The listing builds one solid part. Answer for the finished solid, in the listing's coordinates (mm). Round coordinates to 2 decimals unless told otherwise and drop trailing zeros. Loops run counter-clockwise (first coordinate to the right, second up) from the corner with the lowest first, then second, coordinate; pieces in that order, holes last. Notation, with made-up numbers: (50.5, -15) - (64.5, -15) arc R25 ccw to (64.5, 6) - close; hole circle Ø9 at (55.25, -29.75). An arc over 180 degrees is marked (long way). Write item = value, one per line. Start each with the question number.
1) Section C-C, the plane y = 5.4 is taken. Determine the outline of the cut face in (x, z), and give its area (3 significant figures).
2) Given pin 1 Ø10 at (x, z) = (-14, 16) entering from +Y; pin 2 Ø0.7 at (y, z) = (0.5, 1) entering from -X, each flat-ended and moving along its own axis, determine where each tip first touches the part or whether it passes through.
3) Section B-B, the plane x = -16.75 is taken. Determine the outline of the cut face in (y, z).
4) Section A-A, the plane y = 2.9 is taken. Determine the outline of the cut face in (x, z).
5) Section D-D, the plane x = -9.25 is taken. Determine the outline of the cut face in (y, z), and give its area (3 significant figures).
6) Straight lines are drawn through the part: line 1 along Z through (x, y) = (-11.5, 0.65); line 2 along X through (y, z) = (3.05, 26); line 3 along Y through (x, z) = (2, -10). For each, find the intervals that lie inside material, in ascending order.
from build123d import *

# Parameters (mm, degrees)
BOSS_EXTRUDE1_START       = -15.875
BOSS_EXTRUDE1_DEPTH       = 15.875
BOSS_EXTRUDE1_2_OUTLINE_W = 13.197490677
BOSS_EXTRUDE1_2_OUTLINE_H = 1.397
BOSS_EXTRUDE1_2_DEPTH     = 16.6878
SKETCH2_W                 = 13.197490677
SKETCH2_H                 = 1.397
BOSS_EXTRUDE2_DEPTH       = 16.6878
BOSS_EXTRUDE3_START       = 7.1247
BOSS_EXTRUDE3_DEPTH       = 7.1247
BOSS_EXTRUDE4_DEPTH       = 7.1247
CUT_EXTRUDE1_DEPTH        = 38.210837465
CUT_EXTRUDE2_DEPTH        = 38.210837465
CUT_EXTRUDE3_DEPTH        = 38.210837465
CUT_EXTRUDE4_DEPTH        = 38.210837465
SKETCH9_W                 = 4.6228
SKETCH9_H                 = 4.6228
CUT_EXTRUDE5_DEPTH        = 38.408183622
SKETCH10_W                = 4.6228
SKETCH10_H                = 4.6228
CUT_EXTRUDE6_DEPTH        = 38.408183622
SKETCH11_W                = 4.6228
SKETCH11_H                = 4.6228
CUT_EXTRUDE7_DEPTH        = 38.408183622
SKETCH12_W                = 4.6228
SKETCH12_H                = 4.6228
CUT_EXTRUDE8_DEPTH        = 38.408183622
SKETCH13_W                = 4.6228
SKETCH13_H                = 4.6228
CUT_EXTRUDE9_DEPTH        = 38.210837465
DRAFT1_DEPTH              = 1.397
DRAFT2_DEPTH              = 1.397
CHAMFER1_SIZE             = 2.24506403
SKETCH14_R                = 2.413
CUT_EXTRUDE10_DEPTH       = 2.54
LPATTERN1_COUNT           = 5
LPATTERN1_PITCH           = 12.7


with BuildPart() as part:
    # Boss-Extrude1: read off the stored shape, not the designer's step
    # Boss-Extrude1 outline → Boss-Extrude1 (new body)
    with BuildSketch(Plane.XY.offset(7.9375).offset(BOSS_EXTRUDE1_START)):
        with BuildLine():
            Line((-14.500184662, 2.190749994), (-13.290347173, 1.492249994))
            ThreePointArc((-13.290347173, 1.492249994), (-17.367250005, 5.569152828), (-15.875, -1.1e-08))
            Line((-15.875, -1.1e-08), (3.175, 0))
            Line((3.175, 0), (3.175, 1.397))
            Line((3.175, 1.397), (-15.875, 1.396999989))
            ThreePointArc((-15.875, 1.396999989), (-16.668750005, 4.359315339), (-14.500184662, 2.190749994))
        make_face()
    extrude(amount=BOSS_EXTRUDE1_DEPTH)

    # Boss-Extrude1 2 outline → Boss-Extrude1 2 (add)
    with BuildSketch(Plane.XY.offset(7.9375)):
        with Locations((-3.423745338, 0.6985)):
            Rectangle(BOSS_EXTRUDE1_2_OUTLINE_W, BOSS_EXTRUDE1_2_OUTLINE_H)
    extrude(amount=BOSS_EXTRUDE1_2_DEPTH)

    # Sketch2 → Boss-Extrude2 (add)
    with BuildSketch(Plane(origin=(0, 0, -7.9375), x_dir=(-1, 0, 0), z_dir=(0, 0, -1))):
        with Locations((3.423745338, 0.6985)):
            Rectangle(SKETCH2_W, SKETCH2_H)
    extrude(amount=BOSS_EXTRUDE2_DEPTH)

    # Sketch3 → Boss-Extrude3 (add)
    with BuildSketch(Plane(origin=(0, 0, -24.6253), x_dir=(-1, 0, 0), z_dir=(0, 0, -1)).offset(BOSS_EXTRUDE3_START)):
        with BuildLine():
            Line((15.875, 0), (-3.175, 0))
            Line((-3.175, 0), (-3.175, 1.397))
            Line((-3.175, 1.397), (15.875, 1.397))
            ThreePointArc((15.875, 1.397), (16.668750004, 4.359315344), (14.500184664, 2.190750004))
            Line((14.500184664, 2.190750004), (13.290347175, 1.492250004))
            ThreePointArc((13.290347175, 1.492250004), (17.367250004, 5.569152833), (15.875, 0))
        make_face()
    extrude(amount=-BOSS_EXTRUDE3_DEPTH)

    # Sketch4 → Boss-Extrude4 (add)
    with BuildSketch(Plane.XY.offset(24.6253)):
        with BuildLine():
            Line((-15.875, 1.396999994), (3.175, 1.396999994))
            Line((3.175, 1.396999994), (3.175, -6e-09))
            Line((3.175, -6e-09), (-15.875, -6e-09))
            ThreePointArc((-15.875, -6e-09), (-17.367250004, 5.569152828), (-13.290347175, 1.492249999))
            Line((-13.290347175, 1.492249999), (-14.500184664, 2.190749999))
            ThreePointArc((-14.500184664, 2.190749999), (-16.668750004, 4.359315339), (-15.875, 1.396999994))
        make_face()
    extrude(amount=BOSS_EXTRUDE4_DEPTH)

    # Sketch5 → Cut-Extrude1 (cut, through all)
    with BuildSketch(Plane(origin=(0, 1.397, 0), x_dir=(-1, 0, 0), z_dir=(0, 1, 0))):
        Polygon((-3.175, -16.80493597), (-3.175, -21.29506403), (1.315128061, -16.80493597), align=None)
    extrude(amount=-CUT_EXTRUDE1_DEPTH, mode=Mode.SUBTRACT)

    # Sketch6 → Cut-Extrude2 (cut, through all)
    with BuildSketch(Plane(origin=(0, 1.397, 0), x_dir=(-1, 0, 0), z_dir=(0, 1, 0))):
        Polygon((-3.175, -4.10493597), (-3.175, -8.59506403), (1.315128061, -8.59506403), align=None)
    extrude(amount=-CUT_EXTRUDE2_DEPTH, mode=Mode.SUBTRACT)

    # Sketch7 → Cut-Extrude3 (cut, through all)
    with BuildSketch(Plane(origin=(0, 1.397, 0), x_dir=(-1, 0, 0), z_dir=(0, 1, 0))):
        Polygon((-3.175, 8.59506403), (-3.175, 4.10493597), (1.315128061, 8.59506403), align=None)
    extrude(amount=-CUT_EXTRUDE3_DEPTH, mode=Mode.SUBTRACT)

    # Sketch8 → Cut-Extrude4 (cut, through all)
    with BuildSketch(Plane(origin=(0, 1.397, 0), x_dir=(-1, 0, 0), z_dir=(0, 1, 0))):
        Polygon((-3.175, 21.29506403), (-3.175, 16.80493597), (1.315128061, 16.80493597), align=None)
    extrude(amount=-CUT_EXTRUDE4_DEPTH, mode=Mode.SUBTRACT)

    # Sketch9 → Cut-Extrude5 (cut, through all)
    with BuildSketch(Plane.XZ):
        with Locations((-3.175, 25.4)):
            Rectangle(SKETCH9_W, SKETCH9_H)
    extrude(amount=-CUT_EXTRUDE5_DEPTH, mode=Mode.SUBTRACT)

    # Sketch10 → Cut-Extrude6 (cut, through all)
    with BuildSketch(Plane.XZ):
        with Locations((-3.175, 12.7)):
            Rectangle(SKETCH10_W, SKETCH10_H)
    extrude(amount=-CUT_EXTRUDE6_DEPTH, mode=Mode.SUBTRACT)

    # Sketch11 → Cut-Extrude7 (cut, through all)
    with BuildSketch(Plane.XZ):
        with Locations((-3.175, 0)):
            Rectangle(SKETCH11_W, SKETCH11_H)
    extrude(amount=-CUT_EXTRUDE7_DEPTH, mode=Mode.SUBTRACT)

    # Sketch12 → Cut-Extrude8 (cut, through all)
    with BuildSketch(Plane.XZ):
        with Locations((-3.175, -12.7)):
            Rectangle(SKETCH12_W, SKETCH12_H)
    extrude(amount=-CUT_EXTRUDE8_DEPTH, mode=Mode.SUBTRACT)

    # Sketch13 → Cut-Extrude9 (cut, through all)
    with BuildSketch(Plane(origin=(0, 1.397, 0), x_dir=(-1, 0, 0), z_dir=(0, 1, 0))):
        with Locations((3.175, -25.4)):
            Rectangle(SKETCH13_W, SKETCH13_H)
    extrude(amount=-CUT_EXTRUDE9_DEPTH, mode=Mode.SUBTRACT)

    # Draft1: read off the stored shape, not the designer's step
    # Draft1 outline → Draft1 (add)
    with BuildSketch(Plane(origin=(0, 0, 0), x_dir=(1, 0, 0), z_dir=(0, 1, 0))):
        Polygon((-1.315128061, 16.80493597), (3.175, 16.80493597), (0.92993597, 19.05), align=None)
        Polygon((-1.315128061, 8.59506403), (0.92993597, 6.35), (3.175, 8.59506403), align=None)
    extrude(amount=DRAFT1_DEPTH)

    # Draft2: read off the stored shape, not the designer's step
    # Draft2 outline → Draft2 (add)
    with BuildSketch(Plane(origin=(0, 0, 0), x_dir=(1, 0, 0), z_dir=(0, 1, 0))):
        Polygon((-1.315128061, -8.59506403), (3.175, -8.59506403), (0.92993597, -6.35), align=None)
        Polygon((-1.315128061, -16.80493597), (0.92993597, -19.05), (3.175, -16.80493597), align=None)
    extrude(amount=DRAFT2_DEPTH)

    # Chamfer1
    chamfer1_edges = [part.edges().sort_by_distance(p)[0] for p in [
        (3.175, 0.6985, -31.75),
        (3.175, 0.698499994, 31.75),
    ]]
    chamfer(chamfer1_edges, length=CHAMFER1_SIZE)

    # Sketch14 → Cut-Extrude10 (cut)
    with BuildSketch(Plane(origin=(0, 1.397, 0), x_dir=(1, 0, 0), z_dir=(0, 1, 0))):
        with Locations((-3.175, -25.4)):
            Circle(SKETCH14_R)
    cut_extrude10 = extrude(amount=-CUT_EXTRUDE10_DEPTH, mode=Mode.SUBTRACT)

    # LPattern1: Cut-Extrude10 ×5
    with Locations(*[(0, 0, -i * LPATTERN1_PITCH) for i in range(1, LPATTERN1_COUNT)]):
        add(cut_extrude10, mode=Mode.SUBTRACT)


solid = part.part
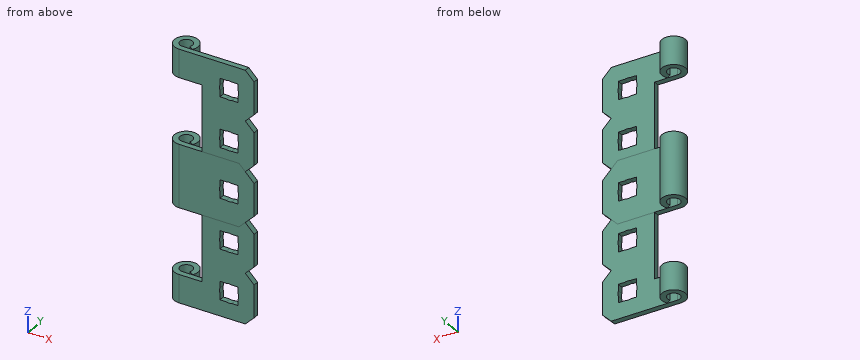
Geometry check:
q1.outline = (-17.63, -31.75) - (-14.12, -31.75) - (-14.12, -24.63) - (-17.63, -24.63) - close; (-17.63, -7.94) - (-14.12, -7.94) - (-14.12, 7.94) - (-17.63, 7.94) - close; (-17.63, 24.63) - (-14.12, 24.63) - (-14.12, 31.75) - (-17.63, 31.75) - close
q1.area = 106 mm2
q2.pin_1 = 1.4
q2.pin_2 = -17.96
q3.outline = (0.13, -31.75) - (1.66, -31.75) - (1.66, -24.63) - (0.13, -24.63) - close; (0.13, -7.94) - (1.66, -7.94) - (1.66, 7.94) - (0.13, 7.94) - close; (0.13, 24.63) - (1.66, 24.63) - (1.66, 31.75) - (0.13, 31.75) - close; (4.31, -31.75) - (5.84, -31.75) - (5.84, -24.63) - (4.31, -24.63) - close; (4.31, -7.94) - (5.84, -7.94) - (5.84, 7.94) - (4.31, 7.94) - close; (4.31, 24.63) - (5.84, 24.63) - (5.84, 31.75) - (4.31, 31.75) - close
q4.outline = (-18.86, -31.75) - (-17.46, -31.75) - (-17.46, -24.63) - (-18.86, -24.63) - close; (-18.86, -7.94) - (-17.46, -7.94) - (-17.46, 7.94) - (-18.86, 7.94) - close; (-18.86, 24.63) - (-17.46, 24.63) - (-17.46, 31.75) - (-18.86, 31.75) - close; (-14.29, -31.75) - (-12.89, -31.75) - (-12.89, -24.63) - (-14.29, -24.63) - close; (-14.29, -7.94) - (-12.89, -7.94) - (-12.89, 7.94) - (-14.29, 7.94) - close; (-14.29, 24.63) - (-12.89, 24.63) - (-12.89, 31.75) - (-14.29, 31.75) - close
q5.outline = (0, -31.75) - (1.4, -31.75) - (1.4, 31.75) - (0, 31.75) - close
q5.area = 88.7 mm2
q6.line_1 = -31.75 to -24.63, -7.94 to 7.94, 24.63 to 31.75
q6.line_2 = -18.86 to -17.46, -14.29 to -12.89
q6.line_3 = 0 to 1.4
